Work out the finished part from the listing and answer in its coordinate system (mm). A direction names the side the tool comes from. Round coordinates to 2 decimals unless told otherwise and drop trailing zeros. Loops run counter-clockwise (first coordinate to the right, second up) from the corner with the lowest first, then second, coordinate; pieces in that order, holes last. Notation, with made-up numbers: (66.5, 80) -> (76.5, 80) arc R8 ccw to (76.5, 91) -> close; hole circle Ø9 at (19.25, 67). An arc over 180 degrees is marked (long way). Use one line per item in the form item = value.
```python
from build123d import *

# Parameters (mm, degrees)
SKETCH_1_W          = 57
SKETCH_1_H          = 57
EXTRUDE_1_DEPTH     = 57
SKETCH_2_R          = 10
CUT_EXTRUDE_1_DEPTH = 52
SKETCH_3_R          = 2.094139209
CUT_EXTRUDE_3_DEPTH = 6
SKETCH_4_R          = 5
EXTRUDE_3_DEPTH     = 11.7
SKETCH_5_R          = 10
EXTRUDE_4_DEPTH     = 26


with BuildPart() as part:
    # 草图1 → 凸台-拉伸1 (new body)
    with BuildSketch(Plane.XY):
        Rectangle(SKETCH_1_W, SKETCH_1_H)
    extrude(amount=EXTRUDE_1_DEPTH)

    # 草图2 → 切除-拉伸1 (cut)
    with BuildSketch(Plane.XY.offset(57)):
        with Locations((28.5, 28.5)):
            Circle(SKETCH_2_R)
        with Locations((-28.5, 28.5)):
            Circle(SKETCH_2_R)
        with Locations((28.5, -28.5)):
            Circle(SKETCH_2_R)
        with Locations((-28.5, -28.5)):
            Circle(SKETCH_2_R)
    extrude(amount=-CUT_EXTRUDE_1_DEPTH, mode=Mode.SUBTRACT)

    # 草图3 → 切除-拉伸3 (cut, through all)
    with BuildSketch(Plane.XY.offset(5)):
        with Locations((23.5, -23.5)):
            Circle(SKETCH_3_R)
        with Locations((-23.5, -23.5)):
            Circle(SKETCH_3_R)
        with Locations((-23.5, 23.5)):
            Circle(SKETCH_3_R)
        with Locations((23.5, 23.5)):
            Circle(SKETCH_3_R)
    extrude(amount=-CUT_EXTRUDE_3_DEPTH, mode=Mode.SUBTRACT)

    # 草图4 → 凸台-拉伸3 (add)
    with BuildSketch(Plane(origin=(0, 0, 0), x_dir=(-1, 0, 0), z_dir=(0, 0, -1))):
        Circle(SKETCH_4_R)
    extrude(amount=EXTRUDE_3_DEPTH)

    # 草图5 → 凸台-拉伸4 (add)
    with BuildSketch(Plane(origin=(0, 0, -11.7), x_dir=(-1, 0, 0), z_dir=(0, 0, -1))):
        Circle(SKETCH_5_R)
    extrude(amount=EXTRUDE_4_DEPTH)


solid = part.part
```
(1) Given P1, Ø6, axis at x = -5.5, z = -27.5, coming from the +Y side; P2, Ø1, axis at y = 5, z = -22.5, coming from the -X side; P3, Ø8, axis at x = 25.5, y = -24, coming from the +Z side; P4, Ø6, axis at x = -22, y = 22, coming from the +Z side, each flat-ended and moving along its own axis, determine where each tip first touches the part or whether it passes through.
Completed:
P1 = 9.68
P2 = -8.93
P3 = 5
P4 = 57
(2) Find section C-C, the plane z = 19.5. Write down the section's boundary in (x, y).
Completed:
outline = (-28.5, -18.5) arc R10 cw to (-18.5, -28.5) -> (18.5, -28.5) arc R10 cw to (28.5, -18.5) -> (28.5, 18.5) arc R10 cw to (18.5, 28.5) -> (-18.5, 28.5) arc R10 cw to (-28.5, 18.5) -> close
(3) For a pull along Z with two mould halves and no side action, classify faces 5 (the cylindrical face through (1.08, -4.88, -5.77)), 6 (the flat face through (26, 25, 5)), 7 (the flat face through (0, 28.5, 28)) as +Z half, -Z half, draft (parallel to the pull), parting line (faces both ways), or undercut.
Completed:
face_5 = undercut
face_6 = +Z half
face_7 = draft
(4) Find section B-B, the plane y = -24.5. Write down the section's boundary in (x, z).
Completed:
outline = (-28.5, 0) -> (-25.34, 0) -> (-25.34, 5) -> (-28.5, 5) -> close; (-21.66, 0) -> (21.66, 0) -> (21.66, 5) -> (19.33, 5) -> (19.33, 57) -> (-19.33, 57) -> (-19.33, 5) -> (-21.66, 5) -> close; (25.34, 0) -> (28.5, 0) -> (28.5, 5) -> (25.34, 5) -> close
(5) Consider L1, parallel to Y at x = -23.5, z = 3.65; L2, parallel to Y at x = 23, z = 2; L3, parallel to Z at x = 9, y = -1. Determine where each line is inside the solid, lowest interval first.
Completed:
L1 = -28.5 to -25.59, -21.41 to 21.41, 25.59 to 28.5
L2 = -28.5 to -25.53, -21.47 to 21.47, 25.53 to 28.5
L3 = -37.7 to -11.7, 0 to 57
(6) For faces 1 (the flat face through (5, -2, -11.7)), 2 (the cylindrical face through (-21.35, -21.51, 31.36)), 3 (the cylindrical face through (-21.51, 21.35, 31.36)), 4 (the flat face through (25, -26, 5)), determine the directions among +Z, -Z, +X, -X, +Y, -Y from which every point of the face is accessible in a straight line to the end or side of a thin tool.
Completed:
face_1 = none
face_2 = +Z, -X, -Y
face_3 = +Z, -X, +Y
face_4 = +Z, +X, -Y
(7) Find section D-D, the plane y = 0. Write down the section's boundary in (x, z).
Completed:
outline = (-28.5, 0) -> (-5, 0) -> (-5, -11.7) -> (-10, -11.7) -> (-10, -37.7) -> (10, -37.7) -> (10, -11.7) -> (5, -11.7) -> (5, 0) -> (28.5, 0) -> (28.5, 57) -> (-28.5, 57) -> close
(8) Find section A-A, the plane x = -8. Write down the section's boundary in (y, z).
Completed:
outline = (-28.5, 0) -> (28.5, 0) -> (28.5, 57) -> (-28.5, 57) -> close; (-6, -37.7) -> (6, -37.7) -> (6, -11.7) -> (-6, -11.7) -> close
